Geometry: final body of the model. Coordinates: model frame, mm. Give positions to 0.01 mm unless a question says otherwise; leave off trailing zeros. Write each loop counter-clockwise with the first axis right and the second up, starting at its lowest first coordinate (ties: lowest second). Pieces come first, ordered by that corner, then holes. Notation, with made-up numbers: (37.25, -8) -> (48.25, -8) arc R20 cw to (48.25, 19) -> close; hole circle Ø4 at (2, -14.5). An arc over 180 degrees is marked (long way). Answer as a JSON object with one key per item and string values. Group by question number.
(1) Section query C-C on y = 0. Output: boundary loops of the cut face in (x, z), plus the area to 3 significant figures.
(2) Contact query for flat-ended pins moving along their axis: pin 1 Ø0.6 at (y, z) = (12, 77) entering from +X; pin 2 Ø0.6 at (x, z) = (-0.5, 76.5) entering from -Y; pin 3 Ø1 at (y, z) = (-5, 77) entering from -X. Output: stop coordinate, or through.
(3) Section query D-D on y = 9. Output: boundary loops of the cut face in (x, z).
(4) Section query B-B on z = 77. State how many separate pieces and enclosed holes the cut face has, plus the area to 3 significant figures.
(5) Material intervals for probe 1 along X at (y, z) = (12, 76.4); probe 2 along X at (y, z) = (7, 77.5); probe 3 along Y at (x, z) = (6.5, 76.55), sorted ascending.
(6) Section query A-A on x = 0. Output: boundary loops of the cut face in (y, z), plus the area to 3 significant figures.
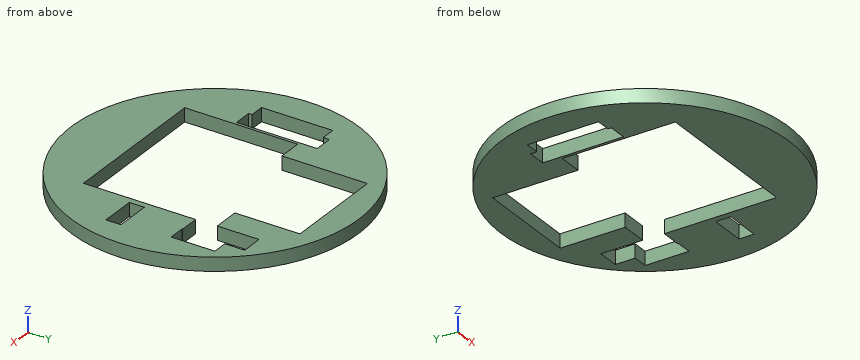
from build123d import *

# Parameters (mm, degrees)
BOX326_W          = 22.5
BOX326_H          = 16.5
BOX326_DEPTH      = 2
BOX327_W          = 15
BOX327_H          = 12.5
BOX327_DEPTH      = 2
BOX319_W          = 2.4
BOX319_H          = 6.4
BOX319_DEPTH      = 2
BOX349_W          = 3.2
BOX349_H          = 9.2
BOX349_DEPTH      = 2
BOX340_W          = 5.2
BOX340_H          = 2.2
BOX340_DEPTH      = 2
BOX339_W          = 2.7
BOX339_H          = 11.8
BOX339_DEPTH      = 2
BOX338_W          = 4
BOX338_H          = 3
BOX338_DEPTH      = 2
BOX320_W          = 2.2
BOX320_H          = 10.4
BOX320_DEPTH      = 2
CYLINDER405_R     = 21
CYLINDER405_DEPTH = 2


with BuildPart() as box326:
    # Box326 → Box326 (new body)
    with BuildSketch(Plane(origin=(-11.5, -12, 76), x_dir=(1, 0, 0), z_dir=(0, 0, 1))):
        with Locations((11.25, 8.25)):
            Rectangle(BOX326_W, BOX326_H)
    extrude(amount=BOX326_DEPTH)


with BuildPart() as box327:
    # Box327 → Box327 (new body)
    with BuildSketch(Plane(origin=(-8, 4.5, 76), x_dir=(1, 0, 0), z_dir=(0, 0, 1))):
        with Locations((7.5, 6.25)):
            Rectangle(BOX327_W, BOX327_H)
    extrude(amount=BOX327_DEPTH)


with BuildPart() as cut_out_narrow_pole:
    # Box319 → Box319 (new body)
    with BuildSketch(Plane(origin=(13.9, 4.3, 76), x_dir=(1, 0, 0), z_dir=(0, 0, 1))):
        with Locations((1.2, 3.2)):
            Rectangle(BOX319_W, BOX319_H)
    extrude(amount=BOX319_DEPTH)


with BuildPart() as box349:
    # Box349 → Box349 (new body)
    with BuildSketch(Plane(origin=(10.9, 4.4, 76), x_dir=(1, 0, 0), z_dir=(0, 0, 1))):
        with Locations((1.6, 4.6)):
            Rectangle(BOX349_W, BOX349_H)
    extrude(amount=BOX349_DEPTH)


with BuildPart() as box340:
    # Box340 → Box340 (new body)
    with BuildSketch(Plane(origin=(11.9, -4.7, 76), x_dir=(1, 0, 0), z_dir=(0, 0, 1))):
        with Locations((2.6, 1.1)):
            Rectangle(BOX340_W, BOX340_H)
    extrude(amount=BOX340_DEPTH)


with BuildPart() as box339:
    # Box339 → Box339 (new body)
    with BuildSketch(Plane(origin=(-14.6, -4.7, 76), x_dir=(1, 0, 0), z_dir=(0, 0, 1))):
        with Locations((1.35, 5.9)):
            Rectangle(BOX339_W, BOX339_H)
    extrude(amount=BOX339_DEPTH)


with BuildPart() as obj1:
    # Box338 → Box338 (new body)
    with BuildSketch(Plane(origin=(7, 4.5, 76), x_dir=(1, 0, 0), z_dir=(0, 0, 1))):
        with Locations((2, 1.5)):
            Rectangle(BOX338_W, BOX338_H)
    extrude(amount=BOX338_DEPTH)


with BuildPart() as cut_outs002:
    # Box320 → Box320 (new body)
    with BuildSketch(Plane(origin=(-16.7, -4.2, 76), x_dir=(1, 0, 0), z_dir=(0, 0, 1))):
        with Locations((1.1, 5.2)):
            Rectangle(BOX320_W, BOX320_H)
    extrude(amount=BOX320_DEPTH)

    # Fusion090: union Box326, Box327, Cut-out narrow pole, Box349, Box340, Box339, obj1
    add(box326.part)
    add(box327.part)
    add(cut_out_narrow_pole.part)
    add(box349.part)
    add(box340.part)
    add(box339.part)
    add(obj1.part)


with BuildPart() as baseplate:
    # Cylinder405 → Cylinder405 (new body)
    with BuildSketch(Plane.XY.offset(76)):
        Circle(CYLINDER405_R)
    extrude(amount=CYLINDER405_DEPTH)

    # Cut228: cut cut-outs002
    add(cut_outs002.part, mode=Mode.SUBTRACT)


solid = baseplate.part
Answer list:
{
 "1": {"outline": "(-21, 76) -> (-16.7, 76) -> (-16.7, 78) -> (-21, 78) -> close; (-11.9, 76) -> (-11.5, 76) -> (-11.5, 78) -> (-11.9, 78) -> close; (11, 76) -> (21, 76) -> (21, 78) -> (11, 78) -> close", "area": "29.4 mm2"},
 "2": {"pin 1": "x = 17.44", "pin 2": "y = -21", "pin 3": "x = -20.51"},
 "3": {"outline": "(-18.97, 76) -> (-8, 76) -> (-8, 78) -> (-18.97, 78) -> close; (7, 76) -> (10.9, 76) -> (10.9, 78) -> (7, 78) -> close; (16.3, 76) -> (18.97, 76) -> (18.97, 78) -> (16.3, 78) -> close"},
 "4": {"separate pieces": "1", "enclosed holes": "3", "area": "706 mm2"},
 "5": {"probe 1": "-17.23 to -8, 7 to 10.9, 14.1 to 17.23", "probe 2": "-19.8 to -14.6, -11.9 to -8, 16.3 to 19.8", "probe 3": "-19.97 to -12, 17 to 19.97"},
 "6": {"outline": "(-21, 76) -> (-12, 76) -> (-12, 78) -> (-21, 78) -> close; (17, 76) -> (21, 76) -> (21, 78) -> (17, 78) -> close", "area": "26.0 mm2"}
}
